```python
from build123d import *

# Parameters (mm, degrees)
SKETCH1_W           = 234.95
SKETCH1_H           = 50.8
SKETCH1_R           = 2.4892
BOSS_EXTRUDE1_DEPTH = 25.4
SKETCH2_W           = 22.225
SKETCH2_H           = 47.625
CUT_EXTRUDE1_DEPTH  = 242.717402146
SKETCH3_R           = 2.4892
CUT_EXTRUDE2_DEPTH  = 242.717402146


with BuildPart() as part:
    # Sketch1 → Boss-Extrude1 (new body)
    with BuildSketch(Plane(origin=(0, 0, 0), x_dir=(0, 0, -1), z_dir=(1, 0, 0))):
        with Locations((117.475, 25.4)):
            Rectangle(SKETCH1_W, SKETCH1_H)
        with Locations((12.7, 25.4)):
            Circle(SKETCH1_R, mode=Mode.SUBTRACT)
        with Locations((12.7, 38.1)):
            Circle(SKETCH1_R, mode=Mode.SUBTRACT)
        with Locations((12.7, 12.7)):
            Circle(SKETCH1_R, mode=Mode.SUBTRACT)
        with Locations((25.4, 12.7)):
            Circle(SKETCH1_R, mode=Mode.SUBTRACT)
        with Locations((25.4, 25.4)):
            Circle(SKETCH1_R, mode=Mode.SUBTRACT)
        with Locations((25.4, 38.1)):
            Circle(SKETCH1_R, mode=Mode.SUBTRACT)
        with Locations((38.1, 12.7)):
            Circle(SKETCH1_R, mode=Mode.SUBTRACT)
        with Locations((38.1, 25.4)):
            Circle(SKETCH1_R, mode=Mode.SUBTRACT)
        with Locations((38.1, 38.1)):
            Circle(SKETCH1_R, mode=Mode.SUBTRACT)
        with Locations((114.3, 12.7)):
            Circle(SKETCH1_R, mode=Mode.SUBTRACT)
        with Locations((114.3, 25.4)):
            Circle(SKETCH1_R, mode=Mode.SUBTRACT)
        with Locations((114.3, 38.1)):
            Circle(SKETCH1_R, mode=Mode.SUBTRACT)
        with Locations((127, 12.7)):
            Circle(SKETCH1_R, mode=Mode.SUBTRACT)
        with Locations((127, 25.4)):
            Circle(SKETCH1_R, mode=Mode.SUBTRACT)
        with Locations((127, 38.1)):
            Circle(SKETCH1_R, mode=Mode.SUBTRACT)
        with Locations((190.5, 12.7)):
            Circle(SKETCH1_R, mode=Mode.SUBTRACT)
        with Locations((190.5, 25.4)):
            Circle(SKETCH1_R, mode=Mode.SUBTRACT)
        with Locations((190.5, 38.1)):
            Circle(SKETCH1_R, mode=Mode.SUBTRACT)
        with Locations((203.2, 12.7)):
            Circle(SKETCH1_R, mode=Mode.SUBTRACT)
        with Locations((203.2, 25.4)):
            Circle(SKETCH1_R, mode=Mode.SUBTRACT)
        with Locations((203.2, 38.1)):
            Circle(SKETCH1_R, mode=Mode.SUBTRACT)
        with Locations((215.9, 12.7)):
            Circle(SKETCH1_R, mode=Mode.SUBTRACT)
        with Locations((215.9, 25.4)):
            Circle(SKETCH1_R, mode=Mode.SUBTRACT)
        with Locations((215.9, 38.1)):
            Circle(SKETCH1_R, mode=Mode.SUBTRACT)
    extrude(amount=BOSS_EXTRUDE1_DEPTH)

    # Sketch2 → Cut-Extrude1 (cut, through all)
    with BuildSketch(Plane.XY):
        with Locations((12.7, 25.4)):
            Rectangle(SKETCH2_W, SKETCH2_H)
    extrude(amount=-CUT_EXTRUDE1_DEPTH, mode=Mode.SUBTRACT)

    # Sketch3 → Cut-Extrude2 (cut, through all)
    with BuildSketch(Plane(origin=(0, 50.8, 0), x_dir=(1, 0, 0), z_dir=(0, 1, 0))):
        with Locations(Location((12.7, 222.25, 0), (0, 0, 270))):
            Circle(SKETCH3_R)
        with Locations(Location((12.7, 209.55, 0), (0, 0, 270))):
            Circle(SKETCH3_R)
        with Locations(Location((12.7, 196.85, 0), (0, 0, 270))):
            Circle(SKETCH3_R)
        with Locations(Location((12.7, 184.15, 0), (0, 0, 270))):
            Circle(SKETCH3_R)
        with Locations(Location((12.7, 171.45, 0), (0, 0, 270))):
            Circle(SKETCH3_R)
        with Locations(Location((12.7, 158.75, 0), (0, 0, 270))):
            Circle(SKETCH3_R)
        with Locations(Location((12.7, 146.05, 0), (0, 0, 270))):
            Circle(SKETCH3_R)
        with Locations(Location((12.7, 133.35, 0), (0, 0, 270))):
            Circle(SKETCH3_R)
        with Locations(Location((12.7, 120.65, 0), (0, 0, 270))):
            Circle(SKETCH3_R)
        with Locations(Location((12.7, 107.95, 0), (0, 0, 270))):
            Circle(SKETCH3_R)
        with Locations(Location((12.7, 95.25, 0), (0, 0, 270))):
            Circle(SKETCH3_R)
        with Locations(Location((12.7, 82.55, 0), (0, 0, 270))):
            Circle(SKETCH3_R)
        with Locations(Location((12.7, 69.85, 0), (0, 0, 270))):
            Circle(SKETCH3_R)
        with Locations(Location((12.7, 57.15, 0), (0, 0, 270))):
            Circle(SKETCH3_R)
        with Locations(Location((12.7, 44.45, 0), (0, 0, 270))):
            Circle(SKETCH3_R)
        with Locations(Location((12.7, 31.75, 0), (0, 0, 270))):
            Circle(SKETCH3_R)
        with Locations(Location((12.7, 19.05, 0), (0, 0, 270))):
            Circle(SKETCH3_R)
    extrude(amount=-CUT_EXTRUDE2_DEPTH, mode=Mode.SUBTRACT)


solid = part.part
```
Work out the finished part from the listing and answer in its coordinate system (mm). A direction names the side the tool comes from. Coordinates: 2 decimals unless noted, no trailing zeros. Write each loop counter-clockwise with the first axis right and the second up, starting at its lowest first coordinate (ties: lowest second). Pieces come first, ordered by that corner, then holes. Notation, with made-up numbers: (72.5, 35.25) - (93.5, 35.25) arc R10 ccw to (93.5, 49.25) - close; hole circle Ø4 at (46.5, 83.25). An arc over 180 degrees is marked (long way). Answer as a JSON object with one key per item and string values.
Q1. Which of the six approach directions +Z, -Z, +X, -X, +Y, -Y give full straight-line access (tool end or side, diameter ignored) to faces 3 (the flat face through (13, 1.587, -116)), 4 (the cylindrical face through (15.17, 0.8, -95.57))?
Results list:
{"face 3": "+Z, -Z", "face 4": "+Y, -Y"}
Q2. Find section B-B (z = -38.1). State how many separate pieces and enclosed holes the cut face has, plus the area to 3 significant figures.
Results list:
{"separate pieces": "6", "enclosed holes": "0", "area": "184 mm^2"}
Q3. Find section A-A (z = -146.05). Write down the section's boundary in (x, y).
Results list:
{"outline": "(0, 0) - (10.21, 0) - (10.21, 1.59) - (1.59, 1.59) - (1.59, 49.21) - (10.21, 49.21) - (10.21, 50.8) - (0, 50.8) - close; (15.19, 0) - (25.4, 0) - (25.4, 50.8) - (15.19, 50.8) - (15.19, 49.21) - (23.81, 49.21) - (23.81, 1.59) - (15.19, 1.59) - close"}
Q4. Find section C-C (x = 20.25). Write down the section's boundary in (y, z).
Results list:
{"outline": "(0, -234.95) - (1.59, -234.95) - (1.59, 0) - (0, 0) - close; (49.21, -234.95) - (50.8, -234.95) - (50.8, 0) - (49.21, 0) - close"}
Q5. For a pull along Y with two mould halves and no side action, classify faces 1 (the cylindrical face through (13.448, 50.017, -143.676)), 2 (the cylindrical face through (24.595, 35.892, -26.549)) as pulls with the +Y half, pulls with the -Y half, needs draft (parallel to the pull), parting line crosses it, or undercut.
Results list:
{"face 1": "needs draft", "face 2": "undercut"}
Q6. Consider L1, parallel to Y at x = 1.1, z = -38.1; L2, parallel to X at y = 14.5, z = -195; L3, parallel to Y at x = 10.5, z = -128. Determine where each line is inside the solid, lowest interval first. Write a range as from..to.
Results list:
{"L1": "y = 0..10.21, 15.19..22.91, 27.89..35.61, 40.59..50.8", "L2": "x = 0..1.59, 23.81..25.4", "L3": "y = 0..1.59, 49.21..50.8"}
